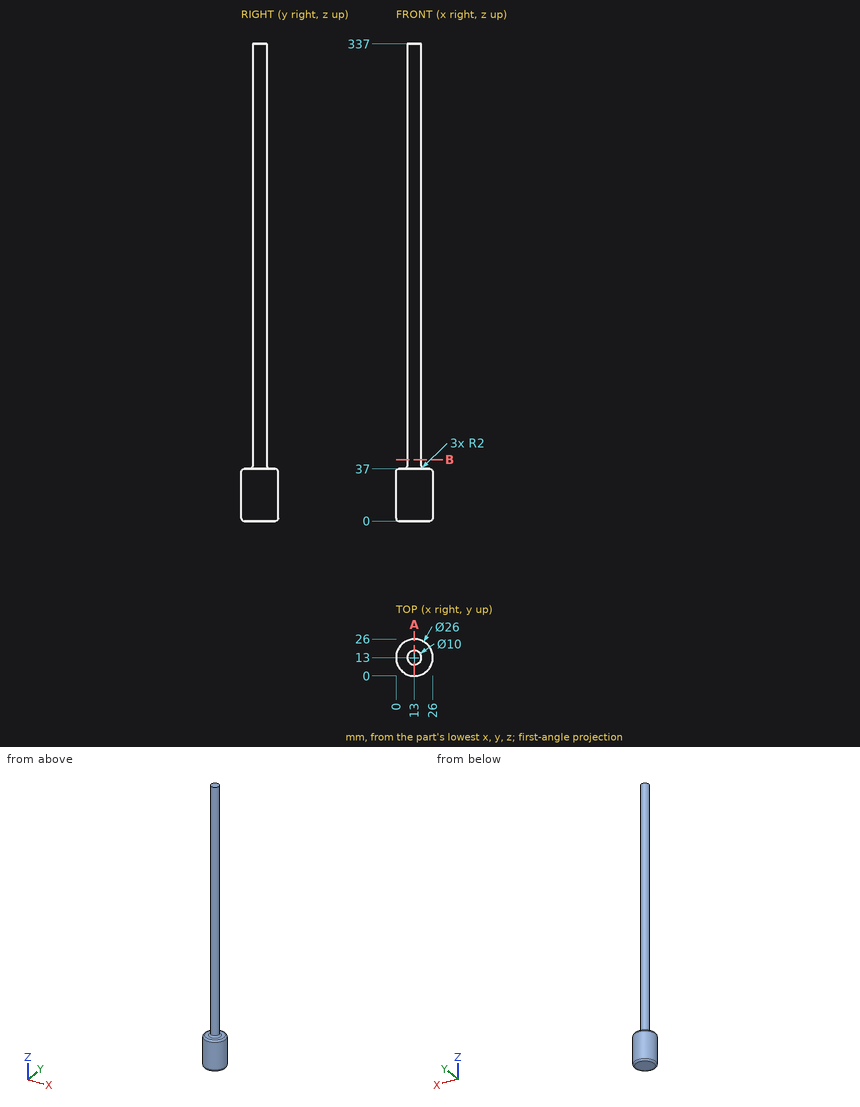
Job drawing, mm, ordinate dimensions from the low corner. One solid piece. Give positions to 0.01 mm unless a question says otherwise; leave off trailing zeros. Order: outer loops, then holes, each group sorted by start corner. A loop starts at its lowest first (then second) coordinate and runs counter-clockwise, first axis right, second up. Notation, with made-up numbers: (85.25, 38.5) - (109.25, 38.5) arc R18 ccw to (109.25, 45.5) - close; hole circle Ø3 at (57.5, -29). An arc over 180 degrees is marked (long way). Answer in a Markdown table with one row per item.
1. Saw through at A-A, the plane x = 13. Give the cut face in (y, z), plus the area to 3 significant figures.
Data:
| item | result |
|---|---|
| outline | (0, 2) arc R2 ccw to (2, 0) - (24, 0) arc R2 ccw to (26, 2) - (26, 35) arc R2 ccw to (24, 37) - (20, 37) arc R2 cw to (18, 39) - (18, 337) - (8, 337) - (8, 39) arc R2 cw to (6, 37) - (2, 37) arc R2 ccw to (0, 35) - close |
| area | 3,960 mm² |
2. Saw through at B-B, the plane z = 43.5. Give the cut face in (x, y).
Data:
| item | result |
|---|---|
| outline | circle Ø10 at (13, 13) |
3. Probe probe 1 along Z at (x, y) = (5.75, 11.5); probe 2 along Z at (x, y) = (13.5, 19.5); probe 3 along X at (y, z) = (16.5, 195.5). List the from-to ranges inside material, lowest first. Write a range as [from, to].
Data:
| item | result |
|---|---|
| probe 1 | z = [0, 37] |
| probe 2 | z = [0, 37.06] |
| probe 3 | x = [9.43, 16.57] |
4. Flat gauge pins, fed straight in: pin 1 (5 mm diameter, centred on x = 15, z = 173.5, fed in from +Y); pin 2 (6 mm diameter, centred on x = 16, z = 264.5, fed in from -Y); pin 3 (2 mm diameter, centred on x = 21, y = 22.5, fed in from -Z). Where does each tip first touch, or does it go through?
Data:
| item | result |
|---|---|
| pin 1 | stops at y = 18 |
| pin 2 | stops at y = 8 |
| pin 3 | stops at z = 0.04 |
